For this review, take the finished solid that the model builds, in its own axes (mm). A direction names the side the tool comes from. Give positions to 0.01 mm unless a question says otherwise; leave off trailing zeros. Order: outer loops, then holes, each group sorted by start corner. A loop starts at its lowest first (then second) coordinate and runs counter-clockwise, first axis right, second up. Notation, with made-up numbers: (22.25, -38.75) - (33.25, -38.75) arc R11 cw to (33.25, -25.75) - close; hole circle Ø4 at (86, -18.5). An arc over 180 degrees is marked (long way). Use a Markdown table: item, result. Add a question column.
1) We need section C-C on z = -10. Write out the cut boundary in (x, y), then the cut area to 3 significant figures.
2) Machinability: for faces 1 (the face through (0, 0, 15)), 2 (the face through (1.5, 0.07, -9.91)), 3 (the face through (1.5, 0.07, 9.78)), which of the approach directions +Z, -Z, +X, -X, +Y, -Y give a long, thin tool a straight path to every point of the face, cutting with its end or side? Answer none if there is none.
3) Mouldability with a two-part tool opening along Z and no side actions: class faces 4 (the face through (-3.233, -1.341, -0.07)), 5 (the face through (0, 2, 5)), 6 (the face through (0, 2, -5)) as released by +Z, released by -Z, zero draft, split by the parting line, or undercut.
4) We need section D-D on y = 3. Write out the cut boundary in (x, z).
5) Clearance check with flat-ended pins moving along their axes: P1, Ø2, axis at x = -0.5, y = 2.5, coming from the +Z side; P2, Ø1, axis at x = -2.5, y = -3, coming from the -Z side; P3, Ø2, axis at y = -1.5, z = 5, coming from the +X side. State where each tip first meets the part, or that it passes through.
6) We need section A-A on y = 0. Write out the cut boundary in (x, z), then the cut area to 3 significant figures.
7) Wall thickness on L1, parallel to Z at x = 2.25, y = 2.5; L2, parallel to Y at x = 0, z = -11.25; L3, parallel to Y at x = -1.25, z = 13.75: over which ranges is each line inside the solid? List them lowest first.
Autodesk Inventor part; units mm, degrees
ref_plane "YZ Plane" through (0, 0, 0) normal (1, 0, 0) x (0, 1, 0)
ref_plane "XZ Plane" through (0, 0, 0) normal (0, 1, 0) x (-1, 0, 0)
ref_plane "XY Plane" through (0, 0, 0) normal (0, 0, 1) x (1, 0, 0)
sketch "Boceto1" plane through (0, 0, 0) normal (0, 1, 0) x (-1, 0, 0)
  line L0 (0, 15) -> (1.5, 15)
  line L1 (1.5, 15) -> (1.5, 5)
  line L2 (1.5, 5) -> (3.5, 5)
  line L3 (3.5, 5) -> (3.5, -5)
  line L4 (3.5, -5) -> (1.5, -5)
  line L5 (1.5, -5) -> (1.5, -15)
  line L6 (1.5, -15) -> (0, -15)
  line L7 (0, -15) -> (0, 15)
  point P0 (0, 0)
  point P1 (0, 0)
  dimension "d0" = 7
  dimension "d1" = 3
  dimension "Dedos" = 10
  dimension "d3" = 30
revolve "Revolución1" add sketch "Boceto1" angle 360 about axis through (0, 0, -15) along (0, 0, 1)
thread "Rosca2"
thread "Rosca3"
chamfer "Chaflán1" distance 0.3067 angle 45 2 edges at (1.5, 0, 15) (1.5, 0, -15)
properties part number "Clavija" material "Aluminio 6061"
Checked values:
| question | item | result |
|---|---|---|
| 1 | outline | circle Ø3 at (0, 0) |
| 1 | area | 7.07 mm² |
| 2 | face 1 | +Z, +X, -X, +Y, -Y |
| 2 | face 2 | -Z |
| 2 | face 3 | +Z |
| 3 | face 4 | zero draft |
| 3 | face 5 | released by +Z |
| 3 | face 6 | released by -Z |
| 4 | outline | (-1.8, -5) - (1.8, -5) - (1.8, 5) - (-1.8, 5) - close |
| 5 | P1 | z = 5 |
| 5 | P2 | z = -5 |
| 5 | P3 | x = 3.46 |
| 6 | outline | (-3.5, -5) - (-1.5, -5) - (-1.5, -14.69) - (-1.19, -15) - (1.19, -15) - (1.5, -14.69) - (1.5, -5) - (3.5, -5) - (3.5, 5) - (1.5, 5) - (1.5, 14.69) - (1.19, 15) - (-1.19, 15) - (-1.5, 14.69) - (-1.5, 5) - (-3.5, 5) - close |
| 6 | area | 130 mm² |
| 7 | L1 | -5 to 5 |
| 7 | L2 | -1.5 to 1.5 |
| 7 | L3 | -0.83 to 0.83 |
